Autodesk Inventor part; units mm, degrees
ref_plane "Work Plane1" through (-49.495, 1.3716, 1.51) normal (0, 0, 1) x (1, 0, 0)
ref_plane "YZ Plane" through (0, 0, 0) normal (1, 0, 0) x (0, 1, 0)
ref_plane "XZ Plane" through (0, 0, 0) normal (0, 1, 0) x (-1, 0, 0)
sketch "Sketch1" plane through (0, 0, 0) normal (0, 0, 1) x (1, 0, 0)
  circle A0 centre (-41.65, 59.825) radius 1.6
  circle A1 centre (-41.15, 6.075) radius 1.6
  circle A2 centre (-7.15, 59.825) radius 1.6
  circle A3 centre (-7.15, 6.075) radius 1.6
  line L0 (-1, 63.5) -> (-1, 0)
  line L1 (-1, 63.5) -> (-49.8, 63.5)
  line L2 (-49.8, 0) -> (-49.8, 63.5)
  line L3 (-1, 0) -> (-49.8, 0)
  ellipse E0 centre (-49.8, 61.0858) end of major axis (-49.8, 63.5) minor radius 1 (-49.8, 63.5) -> (-50.8, 61.0858) ccw
  line L4 (-50.8, 61.0858) -> (-50.8, 1)
  arc A4 (-50.8, 1) -> (-49.8, 0) centre (-49.8, 1) ccw
  arc A5 (-1, 0) -> (0, 1) centre (-1, 1) ccw
  line L5 (0, 1) -> (0, 61.0858)
  ellipse E1 centre (-1, 61.0858) end of major axis (-1, 58.6716) minor radius 1 (0, 61.0858) -> (-1, 63.5) ccw
  line L6 (-48.9, 5.825) -> (-48.9, 59.5)
  arc A6 (-44.9, 63.5) -> (-48.9, 59.5) centre (-44.9, 59.5) ccw
  arc A7 (-1.9, 59.5) -> (-5.9, 63.5) centre (-5.9, 59.5) ccw
  line L7 (-1.9, 59.5) -> (-1.9, 5.825)
  arc A8 (-48.9, 5.825) -> (-44.9, 1.825) centre (-44.9, 5.825) ccw
  line L8 (-5.9, 1.825) -> (-44.9, 1.825)
  arc A9 (-5.9, 1.825) -> (-1.9, 5.825) centre (-5.9, 5.825) ccw
  line L9 (-49.8, 1) -> (-1, 1)
  point P0 (0, 0)
extrude "Extrusion1" add sketch "Sketch1" along normal blind 20 contours E1 L5 A5 L0 | L0 L3 L2 L9 | L2 A4 L4 E0
sketch "Sketch2" plane through (0, 0, 20) normal (0, 0, 1) x (1, 0, 0)
  line L0 (-1, 63.5) -> (-49.8, 63.5)
  ellipse E0 centre (-49.8, 61.0858) end of major axis (-49.8, 63.5) minor radius 1 (-49.8, 63.5) -> (-50.8, 61.0858) ccw
  line L1 (-49.8, 0) -> (-1, 0)
  arc A0 (-1, 0) -> (0, 1) centre (-1, 1) ccw
  line L2 (0, 1) -> (0, 61.0858)
  ellipse E1 centre (-1, 61.0858) end of major axis (-1, 58.6716) minor radius 1 (0, 61.0858) -> (-1, 63.5) ccw
  line L3 (-1, 63.5) -> (-1, 1)
  line L4 (-1, 1) -> (-49.8, 1)
  line L5 (-49.8, 1) -> (-49.8, 63.5)
  ellipse E2 centre (-49.8, 61.0858) end of major axis (-49.8, 63.5) minor radius 1 (-49.8, 63.5) -> (-50.8, 61.0858) ccw
  line L6 (-50.8, 61.0858) -> (-50.8, 1)
  arc A1 (-50.8, 1) -> (-49.8, 0) centre (-49.8, 1) ccw
  arc A2 (-44.9, 63.5) -> (-48.9, 59.5) centre (-44.9, 59.5) ccw
  arc A3 (-1.9, 59.5) -> (-5.9, 63.5) centre (-5.9, 59.5) ccw
  line L7 (-48.9, 59.5) -> (-49.8, 59.5)
  line L8 (-1.9, 59.5) -> (-1, 59.5)
  line L9 (-1.9, 59.5) -> (-48.9, 59.5)
  line L10 (-5.9, 1.825) -> (-44.9, 1.825)
  line L11 (-44.9, 1.825) -> (-49.8, 1.825)
  line L12 (-5.9, 1.825) -> (-1, 1.825)
  point P0 (0, 0)
extrude "Extrusion2" add sketch "Sketch2" along normal blind 2
sketch "Sketch3" plane through (0, 0, 22) normal (0, 0, 1) x (1, 0, 0)
  circle A0 centre (-41.65, 59.825) radius 1.6
  circle A1 centre (-7.15, 59.825) radius 1.6
  circle A2 centre (-7.15, 6.075) radius 1.6
  circle A3 centre (-41.15, 6.075) radius 1.6
  point P0 (0, 0)
extrude "Extrusion3" cut sketch "Sketch3" against normal through all
ref_plane "Work Plane1" through (-49.495, 1.3716, 1.51) normal (0, 0, 1) x (1, 0, 0)
sketch "Sketch4" plane through (0, 0, 22) normal (0, 0, 1) x (1, 0, 0)
  circle A0 centre (-41.65, 59.825) radius 1.6
  circle A1 centre (-41.15, 6.075) radius 1.6
  circle A2 centre (-7.15, 6.075) radius 1.6
  circle A3 centre (-7.15, 59.825) radius 1.6
  circle A4 centre (-41.65, 59.825) radius 2.6
  circle A5 centre (-7.15, 59.825) radius 2.6
  circle A6 centre (-7.15, 6.075) radius 2.6
  circle A7 centre (-41.15, 6.075) radius 2.6
  point P0 (0, 0)
  dimension "d10" = 1
  dimension "d11" = 1
  dimension "d12" = 1
  dimension "d13" = 1
extrude "Extrusion4" add sketch "Sketch4" against normal up to surface (20.49 mm away)
properties part number "case-top"
Work out the finished part from the listing and answer in its coordinate system (mm). A direction names the side the tool comes from. Give positions to 0.01 mm unless a question says otherwise; leave off trailing zeros. Loops run counter-clockwise (first coordinate to the right, second up) from the corner with the lowest first, then second, coordinate; pieces in that order, holes last. Notation, with made-up numbers: (66.5, 67) -> (73.5, 67) arc R23 ccw to (73.5, 97) -> close; hole circle Ø7 at (4.5, 30.25). An arc over 180 degrees is marked (long way). Use CSV: the item, a comma, the result in double quotes.
1. The part is cut by section A-A (x = -7.15). Write down the section's boundary in (y, z) (3 decimals).
Found:
outline,"(0, 0) -> (1, 0) -> (1, 20) -> (3.475, 20) -> (3.475, 1.51) -> (4.475, 1.51) -> (4.475, 22) -> (0, 22) -> close; (7.675, 1.51) -> (8.675, 1.51) -> (8.675, 20) -> (57.225, 20) -> (57.225, 1.51) -> (58.225, 1.51) -> (58.225, 22) -> (7.675, 22) -> close; (61.425, 1.51) -> (62.425, 1.51) -> (62.425, 20) -> (63.5, 20) -> (63.5, 22) -> (61.425, 22) -> close"
2. Flat-ended cylindrical pins translate along their axes: pin 1 Ø2.5 at (x, y) = (-7.15, 6.075) entering from +Z; pin 2 Ø5 at (x, y) = (-7.15, 59.825) entering from -Z; pin 3 Ø3 at (x, y) = (-16.5, 13.5) entering from -Z; pin 4 Ø6 at (x, z) = (-35, 9.5) entering from +Y. Find the tip coordinate at first contact, or state that the pin passes through.
Found:
pin 1,"through"
pin 2,"z = 1.51"
pin 3,"z = 20"
pin 4,"y = 1"
3. The mould has two halves that part along X. Classify faces 1 (the flat face through (-41, 4, 1.51)), 2 (the flat face through (0, 31, 11)), 3 (the flat face through (-50, 32, 0)): +X half, -X half, draft (parallel to the pull), parting line (faces both ways), or undercut.
Found:
face 1,"undercut"
face 2,"+X half"
face 3,"draft"
4. The part is cut by section B-B (y = 26). Write down the section's boundary in (x, z), then the cut area to 3 significant figures.
Found:
outline,"(-50.8, 0) -> (-49.8, 0) -> (-49.8, 20) -> (-1, 20) -> (-1, 0) -> (0, 0) -> (0, 22) -> (-50.8, 22) -> close"
area,"142 mm^2"
5. The part is cut by section C-C (x = -20). Write down the section's boundary in (y, z).
Found:
outline,"(0, 0) -> (1, 0) -> (1, 20) -> (63.5, 20) -> (63.5, 22) -> (0, 22) -> close"
6. The part is cut by section D-D (z = 4). State how many separate pieces and enclosed holes the cut face has, then the cut area to 3 significant figures.
Found:
separate pieces,"5"
enclosed holes,"4"
area,"227 mm^2"
7. Straight lines are drawn through the part: line 1 (Y direction, x = -7.15, z = 10.5) (3 decimals); line 2 (X direction, y = 60, z = 9.75); line 3 (X direction, y = 19, z = 7). For each, find the intervals that lie inside material, in ascending order.
Found:
line 1,"0 to 1, 3.475 to 4.475, 7.675 to 8.675, 57.225 to 58.225, 61.425 to 62.425"
line 2,"-50.8 to -49.8, -44.24 to -43.24, -40.06 to -39.06, -9.74 to -8.74, -5.56 to -4.56, -1 to 0"
line 3,"-50.8 to -49.8, -1 to 0"
8. A tool of negligible diameter and unlimited length cuts with its end or side. For faces 4 (the flat face through (-26, 33, 20)), 5 (the flat face through (-7, 58, 1.51)), 6 (the cylindrical face through (-7.36, 61.41, 11.9)), from which of +Z, -Z, +X, -X, +Y, -Y can it reach the whole face along a straight path? Write none if from no direction.
Found:
face 4,"-Z"
face 5,"-Z, +Y"
face 6,"+Z, -Z"
